from build123d import *

# Parameters (mm, degrees)
F0_W            = 70
F0_H            = 18
F1_DEPTH        = 3.5
F2_W            = 5
F2_H            = 18
F3_DEPTH        = 70
F5_DEPTH        = 3
F8_R            = 5
F9_R            = 1
F11_D           = 4.4
F11_CSINK_D     = 8.4
F11_CSINK_ANGLE = 90


with BuildPart() as f1:
    # F0 (on Front) → F1 (new body)
    with BuildSketch(Plane.XZ):
        Rectangle(F0_W, F0_H)
    extrude(amount=F1_DEPTH)

    # F2 (on face) → F3 (join)
    with BuildSketch(Plane.XZ.offset(3.5)):
        with Locations((32.5, 0)):
            Rectangle(F2_W, F2_H)
    extrude(amount=F3_DEPTH)

    # F4 (on face) → F5 (join)
    with BuildSketch(Plane(origin=(0, 0, -9), x_dir=(1, 0, 0), z_dir=(0, 0, -1))):
        Polygon((13.5421621762, 3.5), (30, 3.5), (30, 32.0058112935), align=None)
    extrude(amount=-F5_DEPTH)

    # F6: F1 across plane


with BuildPart() as f1_1:
    add(f1.part)
    add(f1.part.mirror(Plane.XY))

    # F7: F1 across plane


with BuildPart() as f1_2:
    add(f1_1.part)
    add(f1_1.part.mirror(Plane.YZ))

    # F8
    f8_edges = [f1_2.edges().sort_by_distance(p)[0] for p in [
        (-32.5, -73.5, -9),
        (-32.5, -73.5, 9),
        (32.5, -73.5, -9),
        (32.5, -73.5, 9),
    ]]
    fillet(f8_edges, radius=F8_R)

    # F9
    f9_edges = [f1_2.edges().sort_by_distance(p)[0] for p in [
        (-35, -34.25, -9),
        (35, -34.25, -9),
        (-30, -50.252906, -9),
        (30, -50.252906, -9),
        (-21.771081, -17.752906, -9),
        (0, -3.5, -9),
        (21.771081, -17.752906, 9),
        (-21.771081, -17.752906, 9),
        (0, -3.5, 9),
        (21.771081, -17.752906, 6),
        (21.771081, -17.752906, -6),
        (-21.771081, -17.752906, 6),
        (-21.771081, -17.752906, -6),
        (21.771081, -17.752906, -9),
    ]]
    fillet(f9_edges, radius=F9_R)

    # F11 (through all)
    with Locations(Plane.XZ.offset(3.5)):
        with Locations((-24, 0), (24, 0)):
            CounterSinkHole(F11_D / 2, F11_CSINK_D / 2, counter_sink_angle=F11_CSINK_ANGLE)


solid = f1_2.part
Here's how the part is built. I have some questions about the finished solid (model axes, mm). A direction names the side the tool comes from. Round coordinates to 2 decimals unless told otherwise and drop trailing zeros. Loops run counter-clockwise (first coordinate to the right, second up) from the corner with the lowest first, then second, coordinate; pieces in that order, holes last.
1. For P1, Ø5, axis at x = -2, z = -3, coming from the -Y side; P2, Ø3.5, axis at x = -24, z = 0, coming from the +Y side; P3, Ø5.5, axis at x = 24, z = 0, coming from the -Y side; P4, Ø10, axis at x = -18, z = 6.5, coming from the -Y side, each with a flat end and sliding along its axis, tell me the tip position at first contact or that it passes through.
Answer list:
P1: stops at y = -3.5
P2: passes through
P3: stops at y = -2.05
P4: stops at y = -19.84
2. If I drill on line 1 along X through (y, z) = (-0.5, 0); line 2 along Z through (x, y) = (-25, -5); line 3 along X through (y, z) = (-26, 1), over which ranges is the centre line in solid material (lowest first)?
Answer list:
line 1: x = -35 to -26.2, -21.8 to 21.8, 26.2 to 35
line 2: z = -9 to -6, 6 to 9
line 3: x = -35 to -30, 30 to 35
3. If we section it at A-A on z = 0: Write out the boundary of the cut face in (x, y).
Answer list:
outline: (-35, -72.5) arc R1 ccw to (-34, -73.5) - (-31, -73.5) arc R1 ccw to (-30, -72.5) - (-30, -3.5) - (-28.2, -3.5) - (-26.2, -1.5) - (-26.2, 0) - (-35, 0) - close; (-21.8, -1.5) - (-19.8, -3.5) - (19.8, -3.5) - (21.8, -1.5) - (21.8, 0) - (-21.8, 0) - close; (26.2, -1.5) - (28.2, -3.5) - (30, -3.5) - (30, -72.5) arc R1 ccw to (31, -73.5) - (34, -73.5) arc R1 ccw to (35, -72.5) - (35, 0) - (26.2, 0) - close
4. If we section it at C-C on x = 5: Write out the boundary of the cut face in (y, z), plus the area to 3 significant figures.
Answer list:
outline: (-3.5, -8) arc R1 ccw to (-2.5, -9) - (0, -9) - (0, 9) - (-2.5, 9) arc R1 ccw to (-3.5, 8) - close
area: 62.6 mm2
5. We'd pull the mould along X, two halves only. Please class faces 4 (the face through (32.52, -72, -7.57)), 5 (the face through (0, -3.5, 0)): +X half, -X half, draft (parallel to the pull), parting line (faces both ways), or undercut.
Answer list:
face 4: draft
face 5: undercut
6. Which directions (+Z, -Z, +X, -X, +Y, -Y) give clear straight access to the entire face, cutting with the end or side of a thin tool? Please do faces 1 (the face through (-21.836, -17.264, -8.715)), 2 (the face through (26, -11, 6)), 3 (the face through (-21.886, -17.952, -7.507)).
Answer list:
face 1: -Z, -Y
face 2: -Y
face 3: +Z, -Z, -Y
7. If we section it at B-B on y = -59: Write out the boundary of the cut face in (x, z), plus the area to 3 significant figures.
Answer list:
outline: (-35, -8) arc R1 ccw to (-34, -9) - (-31, -9) arc R1 ccw to (-30, -8) - (-30, 8) arc R1 ccw to (-31, 9) - (-34, 9) arc R1 ccw to (-35, 8) - close; (30, -8) arc R1 ccw to (31, -9) - (34, -9) arc R1 ccw to (35, -8) - (35, 8) arc R1 ccw to (34, 9) - (31, 9) arc R1 ccw to (30, 8) - close
area: 178 mm2
